from build123d import *

# Parameters (mm, degrees)
EXTRUDE_1_DEPTH     = 4
SKETCH_2_R          = 2.05
CUT_EXTRUDE_1_DEPTH = 1051.370094301
FILLET_2_R          = 3
CUT_EXTRUDE_2_DEPTH = 1051.360446107
FILLET_3_R          = 2
SKETCH_4_R          = 1.6
CUT_EXTRUDE_3_DEPTH = 1051.360446107
SKETCH_5_R          = 1.6
CUT_EXTRUDE_4_DEPTH = 1051.360446107


with BuildPart() as part:
    # 草图1 → 凸台-拉伸1 (new body)
    with BuildSketch(Plane.XY):
        Polygon((-33.921923846, 666.196770569), (0, 645), (0, 692.167136134), (-12.725153277, 700.118694416), align=None)
        Polygon((21.196770569, 678.921923846), (0, 645), (84.804809616, 592.008073577), (106.001580185, 625.929997423), align=None)
        Polygon((0, 692.167136134), (0, 645), (21.196770569, 678.921923846), align=None)
        Polygon((0, 1045), (0, 692.167136134), (21.196770569, 678.921923846), (106.001580185, 625.929997423), (60, 1045), align=None)
    extrude(amount=EXTRUDE_1_DEPTH)

    # 草图2 → 切除-拉伸1 (cut, through all)
    with BuildSketch(Plane.XY.offset(4)):
        with Locations((-8.219066797, 688.459141052)):
            Circle(SKETCH_2_R)
        with Locations((-21.467048403, 667.257938648)):
            Circle(SKETCH_2_R)
        with Locations((-4.50608648, 656.659553364)):
            Circle(SKETCH_2_R)
        with Locations((8.741895126, 677.860755767)):
            Circle(SKETCH_2_R)
        with Locations((12.454875443, 646.061168079)):
            Circle(SKETCH_2_R)
        with Locations((25.702857049, 667.262370483)):
            Circle(SKETCH_2_R)
        with Locations((29.415837366, 635.462782794)):
            Circle(SKETCH_2_R)
        with Locations((42.663818972, 656.663985198)):
            Circle(SKETCH_2_R)
        with Locations((46.37679929, 624.86439751)):
            Circle(SKETCH_2_R)
        with Locations((59.624780895, 646.065599913)):
            Circle(SKETCH_2_R)
        with Locations((63.337761213, 614.266012225)):
            Circle(SKETCH_2_R)
        with Locations((76.585742819, 635.467214629)):
            Circle(SKETCH_2_R)
        with Locations((80.298723136, 603.66762694)):
            Circle(SKETCH_2_R)
        with Locations((93.546704742, 624.868829344)):
            Circle(SKETCH_2_R)
    extrude(amount=-CUT_EXTRUDE_1_DEPTH, mode=Mode.SUBTRACT)

    # 圆角2
    fillet_2_edges = [part.edges().sort_by_distance(p)[0] for p in [
        (0, 1045, 2),
        (60, 1045, 2),
        (106.001580185, 625.929997423, 2),
        (84.804809616, 592.008073577, 2),
        (-33.921923846, 666.196770569, 2),
        (-12.725153277, 700.118694416, 2),
        (0, 692.167136134, 2),
    ]]
    fillet(fillet_2_edges, radius=FILLET_2_R)

    # 草图3 → 切除-拉伸2 (cut, through all)
    with BuildSketch(Plane(origin=(0, 0, 0), x_dir=(-1, 0, 0), z_dir=(0, 0, -1))):
        Polygon((-15, 1005.514609624), (-15, 1030), (-39.485390376, 1030), align=None)
        Polygon((-22.071067812, 998.443541812), (-47.25587803, 1023.62835203), (-53.466755162, 967.047854463), align=None)
        Polygon((-15, 926.837288925), (-15, 991.372474001), (-47.267592538, 959.104881463), align=None)
        Polygon((-22.071067812, 919.766221113), (-55.038080192, 952.733233493), (-63.168141984, 878.669146941), align=None)
        Polygon((-15, 828.75719458), (-15, 912.695153301), (-56.96897936, 870.726173941), align=None)
        Polygon((-22.071067812, 821.686126769), (-64.739467014, 864.354525971), (-75.262007489, 768.495187091), align=None)
        Polygon((-15, 701.941730178), (-15, 814.615058957), (-69.194713321, 760.420345636), align=None)
        Polygon((-19.317026748, 691.888302183), (-76.855856505, 753.975374761), (-88.41047261, 648.713925446), align=None)
    extrude(amount=-CUT_EXTRUDE_2_DEPTH, mode=Mode.SUBTRACT)

    # 圆角3
    fillet_3_edges = [part.edges().sort_by_distance(p)[0] for p in [
        (22.071067812, 919.766221113, 2),
        (63.168141984, 878.669146941, 2),
        (55.038080192, 952.733233493, 2),
        (56.96897936, 870.726173941, 2),
        (15, 912.695153301, 2),
        (15, 828.75719458, 2),
        (22.071067812, 998.443541812, 2),
        (53.466755162, 967.047854463, 2),
        (47.25587803, 1023.62835203, 2),
        (47.267592538, 959.104881463, 2),
        (15, 991.372474001, 2),
        (15, 926.837288925, 2),
        (76.855856505, 753.975374761, 2),
        (19.317026748, 691.888302183, 2),
        (88.41047261, 648.713925446, 2),
        (22.071067812, 821.686126769, 2),
        (75.262007489, 768.495187091, 2),
        (64.739467014, 864.354525971, 2),
        (69.194713321, 760.420345636, 2),
        (15, 814.615058957, 2),
        (15, 701.941730178, 2),
        (39.485390376, 1030, 2),
        (15, 1030, 2),
        (15, 1005.514609624, 2),
    ]]
    fillet(fillet_3_edges, radius=FILLET_3_R)

    # 草图4 → 切除-拉伸3 (cut, through all)
    with BuildSketch(Plane(origin=(0, 0, 0), x_dir=(-1, 0, 0), z_dir=(0, 0, -1))):
        with Locations((-35, 1039)):
            Circle(SKETCH_4_R)
        with Locations((-15, 1039)):
            Circle(SKETCH_4_R)
    extrude(amount=-CUT_EXTRUDE_3_DEPTH, mode=Mode.SUBTRACT)

    # 草图5 → 切除-拉伸4 (cut, through all)
    with BuildSketch(Plane(origin=(0, 0, 0), x_dir=(-1, 0, 0), z_dir=(0, 0, -1))):
        with Locations((-60.912093448, 1009.197039366)):
            Circle(SKETCH_5_R)
        with Locations((-58.72978932, 1029.077621569)):
            Circle(SKETCH_5_R)
        with Locations((-64.403780052, 977.388107843)):
            Circle(SKETCH_5_R)
        with Locations((-66.586084179, 957.507525641)):
            Circle(SKETCH_5_R)
    extrude(amount=-CUT_EXTRUDE_4_DEPTH, mode=Mode.SUBTRACT)


solid = part.part
Check sheet for the modelled part. Datum: model origin and axes. Units: mm. A direction names the side the tool comes from. Give positions to 0.01 mm unless a question says otherwise; leave off trailing zeros. Return JSON: item names as keys, results as strings. Group by question number.
1. Thickness scan on L1, parallel to X at y = 716.5, z = 2.5; L2, parallel to X at y = 776.5, z = 3.6; L3, parallel to X at y = 928.5, z = 0.4. Record the ranges inside material, lowest first.
2. Tool access check on faces 4 (the flat face through (95.79, 609.59, 1.97)), 5 (the flat face through (33.75, 1010.12, 1.97)). Record the directions out of +Z, -Z, +X, -X, +Y, -Y that give a thin tool (end or side, any length) a straight path to the whole face; none if there is none.
3. Cross-section at A-A on z = 2.6. State how many separate pieces and enclosed holes the cut face has, plus the area to 3 significant figures.
4. Go/stop test with flat-tipped pins: pin 1 (2 mm diameter, centred on x = 43.5, z = 3.5, fed in from -Y); pin 2 (1 mm diameter, centred on y = 700.5, z = 1, fed in from +X); pin 3 (1.9 mm diameter, centred on x = 66.59, y = 957.51, fed in from +Z); pin 4 (1.5 mm diameter, centred on y = 856.5, z = 3.5, fed in from -X). Record where each tip stops, or that it passes through.
5. Mould release check, pull along Y, two halves, no side actions. Record for faces 1 (the flat face through (20, 822, 4)), 2 (the flat face through (69.85, 817.78, 1.97)), 3 (the flat face through (83.41, 831.74, 1.97)): released by +Y, released by -Y, zero draft, split by the parting line, or undercut.
Return value:
{
 "1": {"L1": "0 to 15, 28.49 to 42.13, 80.97 to 96.06", "L2": "0 to 15, 53.12 to 67.26, 74.38 to 89.47", "L3": "0 to 30.8, 57.7 to 72.79"},
 "2": {"face 4": "+Z, -Z, +X, -Y", "face 5": "+Z, -Z"},
 "3": {"separate pieces": "1", "enclosed holes": "28", "area": "22,800 mm^2"},
 "4": {"pin 1": "y = 617.19", "pin 2": "x = 97.87", "pin 3": "through", "pin 4": "x = 0"},
 "5": {"face 1": "zero draft", "face 2": "undercut", "face 3": "released by +Y"}
}
